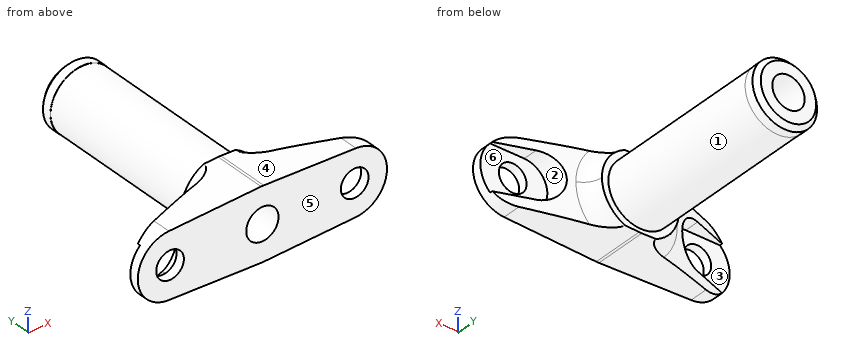
```python
from build123d import *

# Parameters (mm, degrees)
SZKIC1_W                        = 27
SZKIC1_H                        = 25
ZAOKR_GLENIE1_R                 = 4
SZKIC4_R                        = 3
WYTNIJ_WYCI_GNI_CIE3_DEPTH      = 24.0000001
WYTNIJ_WYCI_GNI_CIE3_DEPTH_BACK = 3
WYTNIJ_WYCI_GNI_CIE2_DEPTH      = 24.0000001
SZKIC5_OUTSIDE_W                = 72.072
SZKIC5_OUTSIDE_H                = 72.072
WYTNIJ_WYCI_GNI_CIE4_DEPTH      = 26.0000001
SZKIC8_W                        = 8.35
SZKIC8_H                        = 13.411124978
SZKIC10_R                       = 3.5
WYTNIJ_WYCI_GNI_CIE5_DEPTH      = 52.588875122


with BuildPart() as part:
    # Szkic1 → Obrót1 (revolve)
    with BuildSketch(Plane.XY):
        with Locations((13.5, 12.5)):
            Rectangle(SZKIC1_W, SZKIC1_H)
    revolve(axis=Axis((0, 0, 0), (0, 1, 0)))

    # Szkic2 → Wycięcie-obrót1 (revolve, cut)
    with BuildSketch(Plane.XY):
        Polygon((27, 25), (27, 2), (8.35, 8.788044869), (8.35, 25), align=None)
    revolve(axis=Axis((0, 0, 0), (0, 1, 0)), mode=Mode.SUBTRACT)

    # Zaokrąglenie1
    zaokr_glenie1_edges = [part.edges().sort_by_distance(p)[0] for p in [
        (-8.35, 8.788044869, 0),
    ]]
    fillet(zaokr_glenie1_edges, radius=ZAOKR_GLENIE1_R)

    # Szkic4 → Wytnij-wyciągnięcie3 (cut, two sides)
    with BuildSketch(Plane(origin=(0, 2, 0), x_dir=(1, 0, 0), z_dir=(0, 1, 0))) as wytnij_wyci_gni_cie3_sk:
        with Locations((-20, 0)):
            Circle(SZKIC4_R)
        with Locations((20, 0)):
            Circle(SZKIC4_R)
    extrude(amount=WYTNIJ_WYCI_GNI_CIE3_DEPTH, mode=Mode.SUBTRACT)
    extrude(wytnij_wyci_gni_cie3_sk.sketch, amount=-WYTNIJ_WYCI_GNI_CIE3_DEPTH_BACK, mode=Mode.SUBTRACT)

    # Szkic3 → Wytnij-wyciągnięcie2 (cut, through all)
    with BuildSketch(Plane(origin=(0, 2, 0), x_dir=(1, 0, 0), z_dir=(0, 1, 0))):
        with BuildLine():
            Line((-17.5, 5), (-26.532998323, 5))
            ThreePointArc((-26.532998323, 5), (-27, 0), (-26.532998323, -5))
            Line((-26.532998323, -5), (-17.5, -5))
            ThreePointArc((-17.5, -5), (-12.5, 0), (-17.5, 5))
        make_face()
        with BuildLine():
            Line((17.5, 5), (26.532998323, 5))
            ThreePointArc((26.532998323, 5), (27, 0), (26.532998323, -5))
            Line((26.532998323, -5), (17.5, -5))
            ThreePointArc((17.5, -5), (12.5, 0), (17.5, 5))
        make_face()
    extrude(amount=WYTNIJ_WYCI_GNI_CIE2_DEPTH, mode=Mode.SUBTRACT)

    # Szkic5 outside → Wytnij-wyciągnięcie4 (cut, through all)
    with BuildSketch(Plane.XZ):
        Rectangle(SZKIC5_OUTSIDE_W, SZKIC5_OUTSIDE_H)
        with BuildLine():
            Line((-20.2625, 6.995076393), (-0.290625, 7.744548864))
            ThreePointArc((-0.290625, 7.744548864), (0, 7.75), (0.290625, 7.744548864))
            Line((0.290625, 7.744548864), (20.2625, 6.995076393))
            ThreePointArc((20.2625, 6.995076393), (27, 0), (20.2625, -6.995076393))
            Line((20.2625, -6.995076393), (0.290625, -7.744548864))
            ThreePointArc((0.290625, -7.744548864), (0, -7.75), (-0.290625, -7.744548864))
            Line((-0.290625, -7.744548864), (-20.2625, -6.995076393))
            ThreePointArc((-20.2625, -6.995076393), (-27, 0), (-20.2625, 6.995076393))
        make_face(mode=Mode.SUBTRACT)
    extrude(amount=-WYTNIJ_WYCI_GNI_CIE4_DEPTH, mode=Mode.SUBTRACT)

    # Szkic8 → Wycięcie-obrót2 (revolve, cut)
    with BuildSketch(Plane.XY):
        with Locations((4.175, 18.294437511)):
            Rectangle(SZKIC8_W, SZKIC8_H)
    revolve(axis=Axis((0, 25, 0), (0, -1, 0)), mode=Mode.SUBTRACT)

    # Szkic9 → Obrót2 (revolve)
    with BuildSketch(Plane.XY):
        Polygon((6, 51.588875022), (0, 51.588875022), (0, 11.588875022), (6.95, 11.588875022), (6.95, 48.588875022), (7, 48.588875022), (7, 50.588875022), align=None)
    revolve(axis=Axis((0, 11.588875022, 0), (0, 1, 0)))

    # Szkic10 → Wytnij-wyciągnięcie5 (cut, through all)
    with BuildSketch(Plane(origin=(0, 51.588875022, 0), x_dir=(1, 0, 0), z_dir=(0, 1, 0))):
        Circle(SZKIC10_R)
    extrude(amount=-WYTNIJ_WYCI_GNI_CIE5_DEPTH, mode=Mode.SUBTRACT)


solid = part.part
```
Design review of the part built by this model. Coordinates are the model's own, in mm. Face numbers are marked on the shaded views. A direction names the side the tool comes from. Give positions to 0.01 mm unless a question says otherwise; leave off trailing zeros. Order: outer loops, then holes, each group sorted by start corner. A loop starts at its lowest first (then second) coordinate and runs counter-clockwise, first axis right, second up. Notation, with made-up numbers: (36, 49) -> (45, 49) arc R19 ccw to (45, 83) -> close; hole circle Ø3 at (-6.75, 72.25). An arc over 180 degrees is marked (long way). Write each question's results on one line, items separated by ' | '. Start each with the question number.
Q1. Add section A-A on y = 31. Give the boundary of the cut face in (x, z).
Q2. Add section B-B on z = -1. State how many separate pieces and enclosed holes the cut face has, and give its area (3 significant figures).
Q3. Machinability: for the marked faces 1, 2 and 3, which of the approach directions +Z, -Z, +X, -X, +Y, -Y give a long, thin tool a straight path to every point of the face, cutting with its end or side? Answer none if there is none.
Q4. Wall thickness on L1, parallel to X at y = 1.1, z = 0; L2, parallel to Z at x = 0, y = 21; L3, parallel to Z at x = -20, y = 1.35: over which ranges is each line inside the solid? List them lowest first. Write a range as from..to.
Q5. For pin 1 (2 mm diameter, centred on x = 10, z = -3.5, fed in from +Y); pin 2 (6 mm diameter, centred on y = 9, z = -3, fed in from +X); pin 3 (7 mm diameter, centred on x = -20, z = 0, fed in from +Y); pin 4 (8 mm diameter, centred on x = 0, z = 0, fed in from -Y), all flat-tipped, find the tip position at first contact; note any pin that passes through.
Q6. Mouldability with a two-part tool opening along Z and no side actions: class the marked faces 4, 5 and 6 as +Z half, -Z half, draft (parallel to the pull), parting line (faces both ways), or undercut.
Found:
1) outline: circle Ø13.9 at (0, 0); hole circle Ø7 at (0, 0)
2) separate pieces: 4 | enclosed holes: 0 | area: 502 mm2
3) face 1: none | face 2: +X, +Y | face 3: -X, +Y
4) L1: x = -27..-23, -17..-3.5, 3.5..17, 23..27 | L2: z = -6.95..-3.5, 3.5..6.95 | L3: z = -7..-3, 3..7
5) pin 1: stops at y = 8.69 | pin 2: stops at x = 14.76 | pin 3: stops at y = 2 | pin 4: stops at y = 0
6) face 4: +Z half | face 5: draft | face 6: undercut
